Geometry check sheet. Reference: drawing and pictorial views, mm from the part's lowest x, y, z. A direction names the side the tool comes from. Round coordinates to 2 decimals unless told otherwise and drop trailing zeros. Loops run counter-clockwise (first coordinate to the right, second up) from the corner with the lowest first, then second, coordinate; pieces in that order, holes last. Notation, with made-up numbers: (-14, 42.5) -> (43, 42.5) arc R13 ccw to (43, 46.5) -> close; hole circle Ø1 at (-40, 14.25). An arc over 180 degrees is marked (long way). Use one line per item in the form item = value.
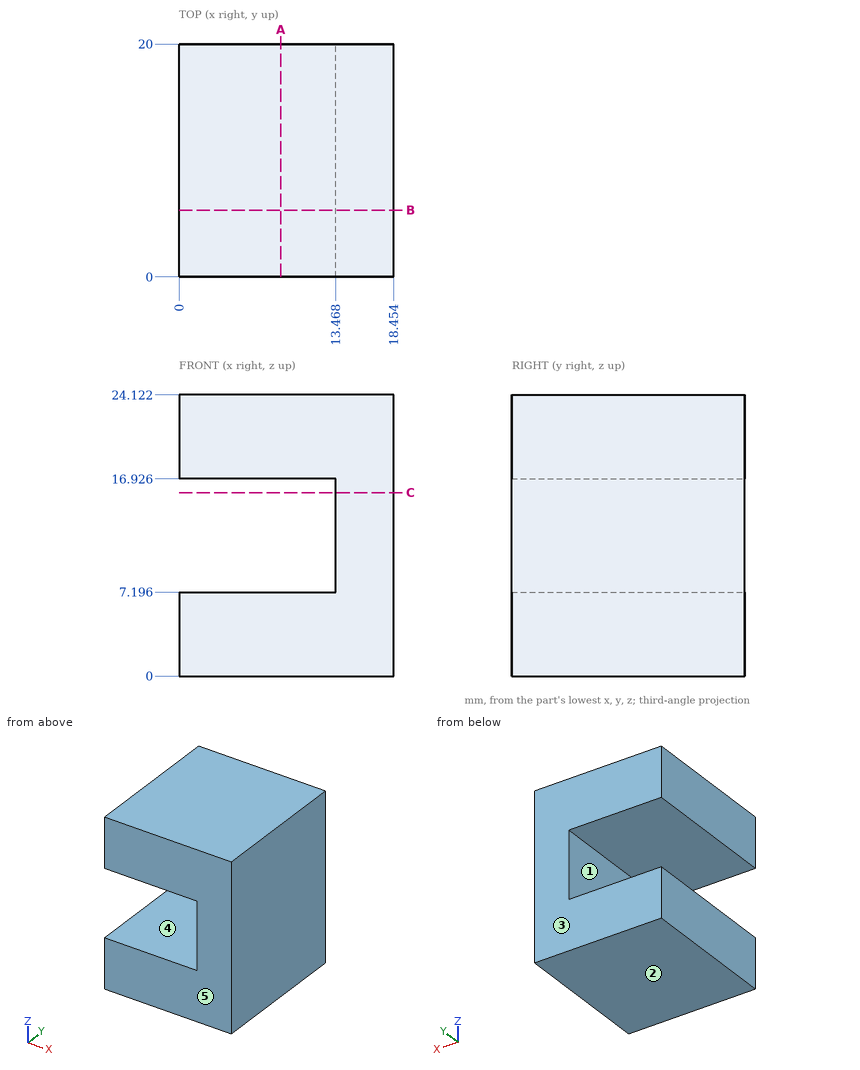
1. Tool access check on the marked faces 4 and 5. Record the directions out of +Z, -Z, +X, -X, +Y, -Y that give a thin tool (end or side, any length) a straight path to the whole face; none if there is none.
Return value:
face_4 = -X, +Y, -Y
face_5 = +Z, -Z, +X, -X, -Y
2. Material ranges on line 1 along Z through (x, y) = (7.25, 16) (1 decimal); line 2 along X through (y, z) = (16.5, 16.25), recorded low to high.
Return value:
line_1 = 0 to 7.2, 16.9 to 24.1
line_2 = 13.47 to 18.45
3. Mould release check, pull along Z, two halves, no side actions. Record for the marked faces 1, 2 and 3: released by +Z, released by -Z, zero draft, split by the parting line, or undercut.
Return value:
face_1 = undercut
face_2 = released by -Z
face_3 = zero draft
4. Section check B-B (y = 5.75). Record the boundary of the cut face in (x, z) (1 decimal).
Return value:
outline = (0, 0) -> (18.5, 0) -> (18.5, 24.1) -> (0, 24.1) -> (0, 16.9) -> (13.5, 16.9) -> (13.5, 7.2) -> (0, 7.2) -> close
5. Section check C-C (z = 15.75). Record the boundary of the cut face in (x, y).
Return value:
outline = (13.47, 0) -> (18.45, 0) -> (18.45, 20) -> (13.47, 20) -> close
6. Section check A-A (x = 8.75). Record the boundary of the cut face in (y, z) (1 decimal), then the cut area to 3 significant figures.
Return value:
outline = (0, 0) -> (20, 0) -> (20, 7.2) -> (0, 7.2) -> close; (0, 16.9) -> (20, 16.9) -> (20, 24.1) -> (0, 24.1) -> close
area = 288 mm2
